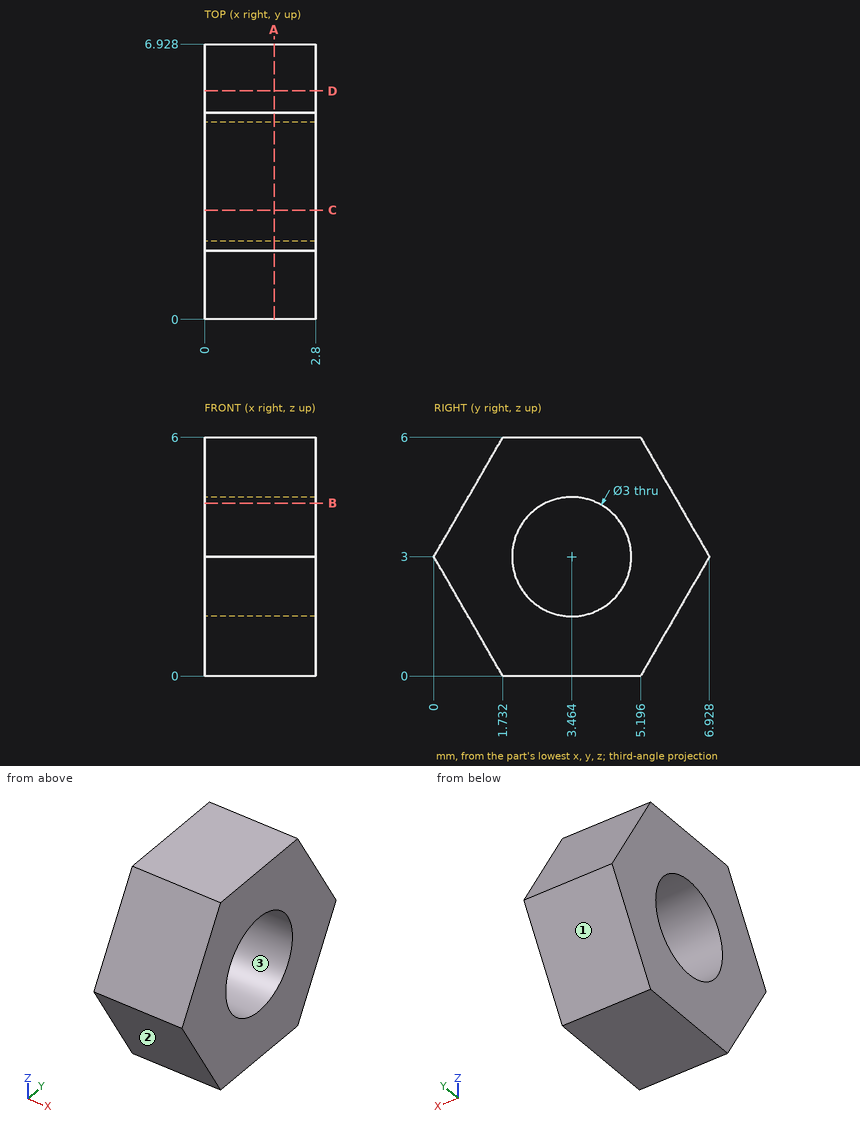
Verification items for this drawing (mm, ordinates from the low corner). Give positions to 0.01 mm unless a question says otherwise; leave off trailing zeros. Write each loop counter-clockwise with the first axis right and the second up, starting at its lowest first coordinate (ties: lowest second). Pieces come first, ordered by that corner, then holes. Notation, with made-up numbers: (84.25, 45) - (112.25, 45) arc R11 cw to (112.25, 54) - close; hole circle Ø9 at (26, -22). An arc over 180 degrees is marked (long way). Answer as a JSON object with one key per item and string values. Group by question number.
1) Release check for a two-part mould opening along Y. For the marked faces 1, 2 and 3 record: pulls with the +Y half, pulls with the -Y half, needs draft (parallel to the pull), parting line crosses it, or undercut.
2) Depth check by flat-ended pin: P1, Ø1.8, axis at y = 3.46, z = 3, coming from the -X side. Enter the tip coordinate at first touch or a pass-through.
3) Sectioned sample at D-D (y = 5.75). Record the cut outline in (x, z).
4) Thickness scan on probe 1 along Z at (x, y) = (0.3, 3.5); probe 2 along Z at (x, y) = (0.5, 2.75); probe 3 along Y at (x, z) = (0.9, 3.1). Record the ranges inside material, lowest first. Write a range as from..to.
5) Sectioned sample at A-A (x = 1.75). Record the cut outline in (y, z).
6) Sectioned sample at C-C (y = 2.75). Record the cut outline in (x, z).
7) Sectioned sample at B-B (z = 4.35). Record the cut outline in (x, y), then the cut area to 3 significant figures.
Geometry results:
{
 "1": {"face 1": "pulls with the +Y half", "face 2": "pulls with the -Y half", "face 3": "undercut"},
 "2": {"P1": "passes through"},
 "3": {"outline": "(0, 0.96) - (2.8, 0.96) - (2.8, 5.04) - (0, 5.04) - close"},
 "4": {"probe 1": "z = 0..1.5, 4.5..6", "probe 2": "z = 0..1.68, 4.32..6", "probe 3": "y = 0.06..1.97, 4.96..6.87"},
 "5": {"outline": "(0, 3) - (1.73, 0) - (5.2, 0) - (6.93, 3) - (5.2, 6) - (1.73, 6) - close; hole circle Ø3 at (3.46, 3)"},
 "6": {"outline": "(0, 0) - (2.8, 0) - (2.8, 1.68) - (0, 1.68) - close; (0, 4.32) - (2.8, 4.32) - (2.8, 6) - (0, 6) - close"},
 "7": {"outline": "(0, 0.78) - (2.8, 0.78) - (2.8, 2.81) - (0, 2.81) - close; (0, 4.12) - (2.8, 4.12) - (2.8, 6.15) - (0, 6.15) - close", "area": "11.4 mm^2"}
}
